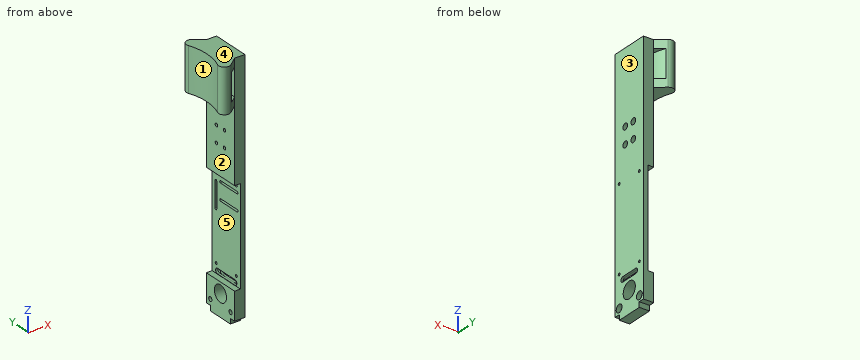
```python
from build123d import *

# Parameters (mm, degrees)
SKETCH022_R         = 7.5
SKETCH022_R_2       = 1.125
PAD002_DEPTH        = 9.4
HOLE007_D           = 4
HOLE007_CBORE_D     = 7.2
HOLE007_CBORE_DEPTH = 4.2
POCKET005_DEPTH     = 5
PAD003_DEPTH        = 40
POCKET006_DEPTH     = 12.5
SKETCH030_W         = 35
SKETCH030_H         = 88.4
POCKET008_DEPTH     = 5.3
POCKET009_DEPTH     = 8
HOLE008_D           = 3
HOLE008_CBORE_D     = 5.7
HOLE008_CBORE_DEPTH = 7.3
SKETCH037_W         = 24.504541
SKETCH037_H         = 35.450562
PAD004_DEPTH        = 0.2
SKETCH038_R         = 4.614907
SKETCH038_R_2       = 4.035565
PAD005_DEPTH        = 0.2


with BuildPart() as part:
    # Sketch022 → Pad002 (new body)
    with BuildSketch(Plane.YZ.offset(62.5)):
        Polygon((-17.5, 225), (-17.5, 4.7), (-12.3, 4.7), (-12.3, 0), (12.3, 0), (12.3, 4.7), (17.5, 4.7), (17.5, 225), align=None)
        with Locations((0, 20)):
            Circle(SKETCH022_R, mode=Mode.SUBTRACT)
        with Locations((-12.5, 114.2)):
            Circle(SKETCH022_R_2, mode=Mode.SUBTRACT)
        with Locations((12.5, 114.2)):
            Circle(SKETCH022_R_2, mode=Mode.SUBTRACT)
        with Locations((-12.5, 38.45)):
            Circle(SKETCH022_R_2, mode=Mode.SUBTRACT)
        with Locations((12.5, 38.45)):
            Circle(SKETCH022_R_2, mode=Mode.SUBTRACT)
        with BuildLine():
            ThreePointArc((-8, 34.7), (-10.3, 32.4), (-8, 30.1))
            Line((-8, 30.1), (8, 30.1))
            ThreePointArc((8, 30.1), (10.3, 32.4), (8, 34.7))
            Line((-8, 34.7), (8, 34.7))
        make_face(mode=Mode.SUBTRACT)
    extrude(amount=PAD002_DEPTH)

    # Hole007 (through all)
    with Locations(Plane.YZ.offset(71.9)):
        with Locations((-12.5, 10), (12.5, 10)):
            CounterBoreHole(HOLE007_D / 2, HOLE007_CBORE_D / 2, HOLE007_CBORE_DEPTH)

    # Sketch026 → Pocket005 (cut)
    with BuildSketch(Plane.YZ.offset(69.9)):
        with BuildLine():
            ThreePointArc((-10.8, 34.75), (-13.15, 32.4), (-10.8, 30.05))
            Line((-10.8, 30.05), (10.8, 30.05))
            ThreePointArc((10.8, 30.05), (13.15, 32.4), (10.8, 34.75))
            Line((-10.8, 34.75), (10.8, 34.75))
        make_face()
    extrude(amount=-POCKET005_DEPTH, mode=Mode.SUBTRACT)

    # Sketch027 → Pad003 (join)
    with BuildSketch(Plane.XY.offset(225)):
        with BuildLine():
            ThreePointArc((46.577049, -18.181818), (50, 0), (46.577049, 18.181818))
            ThreePointArc((54.326085, 23.929844), (48.25594, 24.015802), (46.577049, 18.181818))
            Line((54.326085, 23.929844), (62.5, 17.5))
            Line((62.5, 17.5), (62.5, -17.5))
            Line((62.5, -17.5), (54.326085, -23.929844))
            ThreePointArc((46.577049, -18.181818), (48.25594, -24.015802), (54.326085, -23.929844))
        make_face()
    extrude(amount=-PAD003_DEPTH)

    # Sketch028 → Pocket006 (cut, symmetric)
    with BuildSketch(Plane.XY.offset(205)):
        with BuildLine():
            ThreePointArc((51.961524, -30), (60, 0), (51.961524, 30))
            Line((51.961524, 30), (62.5, 30))
            Line((62.5, 30), (62.5, -30))
            Line((62.5, -30), (51.961524, -30))
        make_face()
    extrude(amount=POCKET006_DEPTH, both=True, mode=Mode.SUBTRACT)

    # Sketch030 → Pocket008 (cut)
    with BuildSketch(Plane.YZ.offset(62.5)):
        with Locations((0, 74)):
            Rectangle(SKETCH030_W, SKETCH030_H)
    extrude(amount=POCKET008_DEPTH, mode=Mode.SUBTRACT)

    # Sketch031 → Pocket009 (cut)
    with BuildSketch(Plane.YZ.offset(62.5)):
        with BuildLine():
            ThreePointArc((13.845935, 107.277863), (12.783162, 108.340636), (11.720389, 107.277863))
            Line((11.720389, 107.277863), (11.720389, 84.030329))
            ThreePointArc((11.720389, 84.030329), (12.783162, 82.967556), (13.845935, 84.030329))
            Line((13.845935, 107.277863), (13.845935, 84.030329))
        make_face()
        with BuildLine():
            ThreePointArc((-13.393928, 109.875952), (-14.456701, 108.813179), (-13.393928, 107.750406))
            Line((-13.393928, 107.750406), (6.990506, 107.750406))
            ThreePointArc((6.990506, 107.750406), (8.053279, 108.813179), (6.990506, 109.875952))
            Line((-13.393928, 109.875952), (6.990506, 109.875952))
        make_face()
        with BuildLine():
            ThreePointArc((-13.495995, 94.718798), (-14.558768, 93.656025), (-13.495995, 92.593252))
            Line((-13.495995, 92.593252), (6.969508, 92.593252))
            ThreePointArc((6.969508, 92.593252), (8.032281, 93.656025), (6.969508, 94.718798))
            Line((-13.495995, 94.718798), (6.969508, 94.718798))
        make_face()
    extrude(amount=POCKET009_DEPTH, mode=Mode.SUBTRACT)

    # Hole008 (through all)
    with Locations(Plane.YZ.offset(71.9)):
        with Locations((-5, 159.1), (5, 159.1), (5, 144.1), (-5, 144.1)):
            CounterBoreHole(HOLE008_D / 2, HOLE008_CBORE_D / 2, HOLE008_CBORE_DEPTH)

    # Sketch037 → Pad004 (join)
    with BuildSketch(Plane.YZ.offset(65.5)):
        with Locations((0.536986, 148.472748)):
            Rectangle(SKETCH037_W, SKETCH037_H)
    extrude(amount=-PAD004_DEPTH)

    # Sketch038 → Pad005 (join)
    with BuildSketch(Plane.YZ.offset(67.7)):
        with Locations((-12.580344, 9.907605)):
            Circle(SKETCH038_R)
        with Locations((12.421253, 10.075215)):
            Circle(SKETCH038_R_2)
    extrude(amount=-PAD005_DEPTH)


solid = part.part
```
Input: part model. Units: mm. Frame: model coordinates. Face numbers are marked on the shaded views. A direction names the side the tool comes from. Give positions to 0.01 mm unless a question says otherwise; leave off trailing zeros. Order: outer loops, then holes, each group sorted by start corner. A loop starts at its lowest first (then second) coordinate and runs counter-clockwise, first axis right, second up. Notation, with made-up numbers: (87, 43) - (129, 43) arc R7 cw to (129, 48) - close; hole circle Ø2 at (-25, -11.5). An arc over 180 degrees is marked (long way). Use a Markdown table: item, result.
(1) Section query C-C (z = 130). Output: boundary loops of the cut face in (x, y), then the cut area to 3 significant figures.
Computed values:
| item | result |
|---|---|
| outline | (62.5, -17.5) - (71.9, -17.5) - (71.9, 17.5) - (62.5, 17.5) - close |
| area | 329 mm2 |
(2) Pin query (flat end, axial travel): pin 1 (1.1 mm diameter, centred on y = 13, z = 97, fed in from -X); pin 2 (3.5 mm diameter, centred on y = -12.5, z = 38.45, fed in from +X); pin 3 (8 mm diameter, centred on x = 59, z = 187.5, fed in from -Y); pin 4 (2 mm diameter, centred on x = 67.5, z = 33, fed in from +Y). Return the tip coordinate at first contact, or that it passes through.
Computed values:
| item | result |
|---|---|
| pin 1 | stops at x = 70.5 |
| pin 2 | stops at x = 71.9 |
| pin 3 | stops at y = -23.4 |
| pin 4 | stops at y = 17.5 |
(3) Line query: line 1 (Z direction, x = 64.5, y = -0.5); line 2 (Z direction, x = 63.7, y = 12.5); line 3 (Z direction, x = 69, y = 15.5). Output: solid intervals per line, ascending. Write a range as from..to.
Computed values:
| item | result |
|---|---|
| line 1 | z = 0..12.52, 27.48..29.8, 118.2..225 |
| line 2 | z = 4.7..8, 12..29.8, 118.2..225 |
| line 3 | z = 4.7..8.01, 11.99..225 |
(4) Draft query along Z for the marked faces 3, 4 and 5. Return one class per face: released by +Z, released by -Z, zero draft, split by the parting line, or undercut.
Computed values:
| item | result |
|---|---|
| face 3 | zero draft |
| face 4 | released by +Z |
| face 5 | undercut |
(5) Section query A-A (y = 0). State how many separate pieces and enclosed holes the cut face has, then the cut area to 3 significant figures.
Computed values:
| item | result |
|---|---|
| separate pieces | 3 |
| enclosed holes | 1 |
| area | 1,910 mm2 |
(6) Access query for the marked faces 1 and 2. Directions: +Z, -Z, +X, -X, +Y, -Y. A direction counts if a zero-diameter tool reaches every point of the face in a straight line with its end or side. Return the directions, or none.
Computed values:
| item | result |
|---|---|
| face 1 | +Z, -Z, -X |
| face 2 | -Z, -X, +Y, -Y |
(7) Section query B-B (z = 20). Output: boundary loops of the cut face in (x, y).
Computed values:
| item | result |
|---|---|
| outline | (62.5, -17.5) - (71.9, -17.5) - (71.9, -7.5) - (62.5, -7.5) - close; (62.5, 7.5) - (71.9, 7.5) - (71.9, 17.5) - (62.5, 17.5) - close |
